Autodesk Inventor part; units mm, degrees
ref_plane "YZ Plane" through (0, 0, 0) normal (1, 0, 0) x (0, 1, 0)
ref_plane "XZ Plane" through (0, 0, 0) normal (0, 1, 0) x (-1, 0, 0)
ref_plane "XY Plane" through (0, 0, 0) normal (0, 0, 1) x (1, 0, 0)
sketch "Sketch1" plane through (0, 0, 0) normal (1, 0, 0) x (0, 1, 0)
  line L0 (0, 0) -> (50.8, 0)
  line L1 (0, 133.35) -> (0, 184.15)
  line L2 (29.2989, 184.15) -> (73.025, 184.15)
  line L3 (73.025, 184.15) -> (73.025, 133.35)
  line L4 (69.85, 180.975) -> (41.9989, 180.975)
  line L5 (3.175, 180.975) -> (3.175, 136.525)
  line L6 (69.85, 136.525) -> (69.85, 180.975)
  line L7 (29.2989, 148.3694) -> (29.2989, 120.4477)
  line L8 (41.9989, 148.9666) -> (41.9989, 122.6874)
  line L9 (0, 133.35) -> (29.2989, 133.35)
  line L10 (41.9989, 133.35) -> (73.025, 133.35)
  line L11 (3.175, 136.525) -> (29.2989, 136.525)
  line L12 (41.9989, 136.525) -> (69.85, 136.525)
  line L13 (35.6489, 182.5625) -> (29.2989, 182.5625)
  line L14 (29.2989, 182.5625) -> (29.2989, 184.15)
  line L15 (35.6489, 182.5625) -> (41.9989, 182.5625)
  line L16 (41.9989, 182.5625) -> (41.9989, 180.975)
  line L17 (35.6489, 170.4093) -> (35.6489, 182.5625)
  line L18 (35.6489, 184.15) -> (35.6489, 196.0777)
  point P0 (3.175, 180.975)
  point P1 (69.85, 136.525)
  dimension "d0" = 50.8
  dimension "d3" = 50.8
  dimension "d4" = 73.025
  dimension "d5" = 3.175
  dimension "d6" = 3.175
  dimension "d7" = 3.175
  dimension "d8" = 3.175
  dimension "d9" = 3.175
  dimension "d11" = 3.175
  dimension "d13" = 26.1239
  dimension "d14" = 12.7
  dimension "d16" = 133.35
  dimension "d17" = 3.175
  dimension "d18" = 3.175
  dimension "d19" = 6.35
  dimension "d20" = 1.5875
  dimension "d21" = 6.35
  dimension "d22" = 6.35
revolve "Revolution1" add sketch "Sketch1" angle 180 about axis through (0, 0, 0) along (0, 1, 0)
sketch "Sketch2" plane through (0, 73.025, 184.15) normal (0, 1, 0) x (1, 0, 0)
  line L0 (0, 184.15) -> (255.0466, 184.15)
  line L1 (255.0466, 184.15) -> (255.0466, -9.3169)
  line L2 (255.0466, -9.3169) -> (0, -9.3169)
  line L3 (0, -9.3169) -> (0, 184.15)
extrude "Extrusion1" cut sketch "Sketch2" against normal through all
properties part number "Outer_Shell_Top_Quarter"
Input: part model. Units: mm. Frame: model coordinates. A direction names the side the tool comes from. Coordinates: 2 decimals unless noted, no trailing zeros. Loops run counter-clockwise (first coordinate to the right, second up) from the corner with the lowest first, then second, coordinate; pieces in that order, holes last. Notation, with made-up numbers: M 3.5,9 L 26.5,9 A18 cw 26.5,22 Z; hole C -31.75,3 d8. An arc over 180 degrees is marked long. Use a Markdown table: item, result. Add a question column.
1) Draft query along Z for faces 4 (the cylindrical face through (97.593, 56.119, -95.47)), 5 (the flat face through (98.92, 41.999, -93.86)), 6 (the cylindrical face through (131.64, 51.47, -128.77)), 7 (the flat face through (98, 69.85, -98)). Return one class per face: +Z half, -Z half, draft (parallel to the pull), parting line (faces both ways), or undercut.
2) Section C-C, the plane x = 16.5. Return the cut outline in (y, z) (3 decimals).
3) Line query: L1, parallel to Y at x = 13, z = -148 (3 decimals); L2, parallel to Z at x = 26, y = 67; L3, parallel to X at y = 47, z = -115.5. Output: solid intervals per line, ascending. Write a range as from..to.
4) Section B-B, the plane z = -52.5. Return the cut outline in (x, y) (3 decimals).
5) Section A-A, the plane y = 61. Return the cut outline in (x, z) (3 decimals), plus the area to 3 significant figures.
6) Set-up query: faces 1 (the cylindrical face through (127.664, 35.56, -130.503)), 2 (the flat face through (161, 71, 0)), 3 (the cylindrical face through (126.55, 55.73, -129.37)). Return all of +Z, -Z, +X, -X, +Y, -Y with unobstructed straight access to the full face (end or side cutting, diameter ignored); none if empty.
7) Pin query (flat end, axial travel): P1, Ø4, axis at x = 123, y = 34, coming from the +Z side; P2, Ø6, axis at x = 41, y = 39.5, coming from the -Z side; P3, Ø8, axis at x = 66, y = 58.5, coming from the -Z side. Return the tip coordinate at first contact, or that it passes through.
Answer below:
| question | item | result |
|---|---|---|
| 1 | face 4 | undercut |
| 1 | face 5 | draft |
| 1 | face 6 | -Z half |
| 1 | face 7 | undercut |
| 2 | outline | M 29.299,-183.409 L 73.025,-183.409 L 73.025,-132.325 L 41.999,-132.325 L 41.999,-135.524 L 69.85,-135.524 L 69.85,-180.221 L 41.999,-180.221 L 41.999,-181.815 L 29.299,-181.815 Z |
| 3 | L1 | 69.85..73.025 |
| 3 | L2 | -182.31..-179.1, -134.03..-130.79 |
| 3 | L3 | 66.65..72.79, 139.33..143.43 |
| 4 | outline | M 122.58,41.999 L 126.027,41.999 L 126.027,69.85 L 173.193,69.85 L 173.193,41.999 L 174.851,41.999 L 174.851,29.299 L 176.508,29.299 L 176.508,73.025 L 122.58,73.025 Z |
| 5 | outline | M 0,-184.15 A184.15 ccw 184.15,0 L 180.975,0 A180.975 cw 0,-180.975 Z; M 0,-136.525 A136.525 ccw 136.525,0 L 133.35,0 A133.35 cw 0,-133.35 Z |
| 5 | area | 1,580 mm2 |
| 6 | face 1 | +Z, -X, -Y |
| 6 | face 2 | +Z, +X, -X, +Y, -Y |
| 6 | face 3 | -Y |
| 7 | P1 | z = -133.06 |
| 7 | P2 | z = -180.19 |
| 7 | P3 | z = -173.4 |
